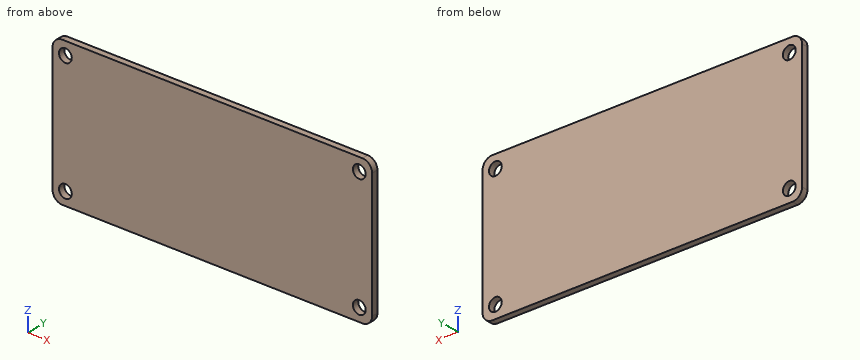
```python
from build123d import *

# Parameters (mm, degrees)
ESBO_O1_W                = 100
ESBO_O1_H                = 45
RESSALTO_EXTRUS_O1_DEPTH = 2
ESBO_O5_R                = 2
CORTE_EXTRUS_O3_DEPTH    = 55.865745233
FILETE1_R                = 3


with BuildPart() as part:
    # Esboço1 → Ressalto-extrusão1 (new body)
    with BuildSketch(Plane(origin=(0, 0, 0), x_dir=(1, 0, 0), z_dir=(0, 1, 0))):
        Rectangle(ESBO_O1_W, ESBO_O1_H)
    extrude(amount=RESSALTO_EXTRUS_O1_DEPTH)

    # Esboço5 → Corte-extrusão3 (cut, through all)
    with BuildSketch(Plane(origin=(0, 2, 0), x_dir=(1, 0, 0), z_dir=(0, 1, 0))):
        with Locations(Location((46, 18.5, 0), (0, 0, 270))):
            Circle(ESBO_O5_R)
        with Locations(Location((46, -18.5, 0), (0, 0, 90))):
            Circle(ESBO_O5_R)
        with Locations(Location((-46, -18.5, 0), (0, 0, 270))):
            Circle(ESBO_O5_R)
        with Locations(Location((-46, 18.5, 0), (0, 0, 90))):
            Circle(ESBO_O5_R)
    extrude(amount=-CORTE_EXTRUS_O3_DEPTH, mode=Mode.SUBTRACT)

    # Filete1
    filete1_edges = [part.edges().sort_by_distance(p)[0] for p in [
        (-50, 1, -22.5),
        (50, 1, -22.5),
        (50, 1, 22.5),
        (-50, 1, 22.5),
    ]]
    fillet(filete1_edges, radius=FILETE1_R)


solid = part.part
```
Geometry: final body of the model. Coordinates: model frame, mm. Coordinates: 2 decimals unless noted, no trailing zeros. Order: outer loops, then holes, each group sorted by start corner. A loop starts at its lowest first (then second) coordinate and runs counter-clockwise, first axis right, second up. Notation, with made-up numbers: M 3.25,26 L 34.25,26 A20 cw 34.25,59 Z; hole C 73,-15 d8. An arc over 180 degrees is marked long. Answer in a Markdown table with one row per item. Add a question column.
Q1. Section query B-B on z = -18.5. Return the cut outline in (x, y).
Q2. Contact query for flat-ended pins moving along their axis: P1, Ø2.5, axis at x = 46, z = 18.5, coming from the -Y side; P2, Ø1.5, axis at x = 6, z = 2, coming from the -Y side. Output: stop coordinate, or through.
Q3. Line query: L1, parallel to X at y = 0.4, z = -18.5; L2, parallel to X at y = 0.1, z = -17. Output: solid intervals per line, ascending.
Q4. Section query A-A on x = 46. Return the cut outline in (y, z).
Completed:
| question | item | result |
|---|---|---|
| 1 | outline | M -50,0 L -48,0 L -48,2 L -50,2 Z; M -44,0 L 44,0 L 44,2 L -44,2 Z; M 48,0 L 50,0 L 50,2 L 48,2 Z |
| 2 | P1 | passes through |
| 2 | P2 | stops at y = 0 |
| 3 | L1 | x = -50 to -48, -44 to 44, 48 to 50 |
| 3 | L2 | x = -50 to -47.32, -44.68 to 44.68, 47.32 to 50 |
| 4 | outline | M 0,-22.5 L 2,-22.5 L 2,-20.5 L 0,-20.5 Z; M 0,-16.5 L 2,-16.5 L 2,16.5 L 0,16.5 Z; M 0,20.5 L 2,20.5 L 2,22.5 L 0,22.5 Z |
